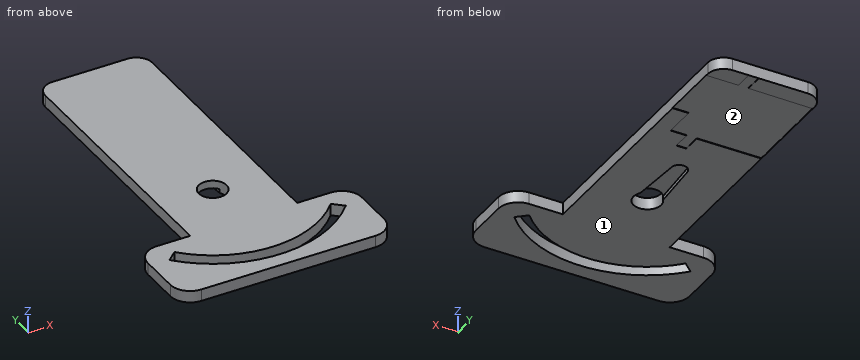
```python
from build123d import *

# Parameters (mm, degrees)
CORTE_EXTERIOR_R        = 3.500001168
SALIENTE_EXTRUIR1_DEPTH = 3
CORTAR_EXTRUIR1_DEPTH   = 1
CORTAR_EXTRUIR2_DEPTH   = 0.1


with BuildPart() as part:
    # Corte exterior → Saliente-Extruir1 (new body)
    with BuildSketch(Plane.XY):
        with BuildLine():
            Line((19.521996462, -6.085833738), (11.021996462, -6.085833738))
            ThreePointArc((11.021996462, -6.085833738), (7.486462556, -7.550299832), (6.021996462, -11.085833738))
            Line((6.021996462, -11.085833738), (6.021996462, -21.085833738))
            ThreePointArc((6.021996462, -21.085833738), (7.486462556, -24.621367644), (11.021996462, -26.085833738))
            Line((11.021996462, -26.085833738), (55.021996462, -26.085833738))
            ThreePointArc((55.021996462, -26.085833738), (58.557530368, -24.621367644), (60.021996462, -21.085833738))
            Line((60.021996462, -21.085833738), (60.021996462, -11.085833738))
            ThreePointArc((60.021996462, -11.085833738), (58.557530368, -7.550299832), (55.021996462, -6.085833738))
            Line((55.021996462, -6.085833738), (46.514841363, -6.085833738))
            Line((46.514841363, -6.085833738), (46.521996462, 58.812041738))
            ThreePointArc((46.521996462, 58.812041738), (45.350423587, 61.640468863), (42.521996462, 62.812041738))
            Line((42.521996462, 62.812041738), (23.521996462, 62.812041738))
            ThreePointArc((23.521996462, 62.812041738), (20.693569337, 61.640468863), (19.521996462, 58.812041738))
            Line((19.521996462, 58.812041738), (19.521996462, -6.085833738))
        make_face()
        with Locations((33.021996462, 7.812041474)):
            Circle(CORTE_EXTERIOR_R, mode=Mode.SUBTRACT)
        with BuildLine():
            Line((55.29494797, -12.330366391), (52.77320204, -10.049840692))
            ThreePointArc((52.77320204, -10.049840692), (33.021996462, -18.817961696), (13.270789317, -10.049842109))
            Line((13.270789317, -10.049842109), (10.749043386, -12.330367808))
            ThreePointArc((10.749043386, -12.330367808), (33.021996462, -22.217961696), (55.29494797, -12.330366391))
        make_face(mode=Mode.SUBTRACT)
    extrude(amount=SALIENTE_EXTRUIR1_DEPTH)

    # Grabado Superficie → Cortar-Extruir1 (cut)
    with BuildSketch(Plane.XY):
        with BuildLine():
            Line((35.89134848, 9.816243852), (35.017032688, 22.202862127))
            ThreePointArc((35.017032688, 22.202862127), (33.021996462, 24.062041474), (31.026960236, 22.202862127))
            Line((31.026960236, 22.202862127), (30.152644444, 9.816243852))
            ThreePointArc((30.152644444, 9.816243852), (33.021996462, 11.312042642), (35.89134848, 9.816243852))
        make_face()
    extrude(amount=CORTAR_EXTRUIR1_DEPTH, mode=Mode.SUBTRACT)

    # grabado linea medio → Cortar-Extruir2 (cut)
    with BuildSketch(Plane.XY):
        Polygon((42.460122518, 43.017187336), (46.540121977, 43.015086813), (46.547921712, 58.165084805), (38.407922791, 58.169275554), (38.41031162, 62.809274939), (35.890311954, 62.810572321), (35.887922498, 58.169356436), (19.547821697, 57.977768849), (19.535965697, 34.948988401), (35.875963531, 34.940576014), (35.873574702, 30.300576629), (38.393574368, 30.299279247), (38.395963198, 34.939278632), (42.455962659, 34.937188407), align=None)
    extrude(amount=CORTAR_EXTRUIR2_DEPTH, mode=Mode.SUBTRACT)


solid = part.part
```
Could you check a few things on this model? Use its own coordinates, in mm. Face numbers are marked on the shaded views. Coordinates: 2 decimals unless noted, no trailing zeros. Write each loop counter-clockwise with the first axis right and the second up, starting at its lowest first coordinate (ties: lowest second). Pieces come first, ordered by that corner, then holes. Notation, with made-up numbers: M -20.75,-39 L 36.25,-39 A24 cw 36.25,-1 Z; hole C 9,41 d4. An arc over 180 degrees is marked long. Answer as CSV lines item,"result". Start each with the question number.
1) We'd pull the mould along X, two halves only. Please class the marked faces 1 and 2: +X half, -X half, draft (parallel to the pull), parting line (faces both ways), or undercut.
2) For P1, Ø1.5, axis at y = -7.5, z = 2.5, coming from the +X side; P2, Ø0.9, axis at x = 17, z = 1.5, coming from the +Y side; P3, Ø4, axis at x = 29.5, y = 52, coming from the -Z side, each with a flat end and sliding along its axis, tell me the tip position at first contact or that it passes through.
3) Please list where these lines run through material, in increasing order: line 1 (X direction, y = -11, z = 1.55); line 2 (Y direction, x = 31.5, z = 1.75); line 3 (X direction, y = -14, z = 1.25). Write a range as from..to.
4) I want a section at A-A, the plane z = 0.55. Please give me the cut outline in (x, y).
5) I want a section at B-B, the plane y = 6. Please give me the cut outline in (x, z).
6) I want a section at D-D, the plane y = 16. Please give me the cut outline in (x, z).
7) I want a section at C-C, the plane y = -14. Please give me the cut outline in (x, z), and give its area (3 significant figures).
Data:
1,face 1,"draft"
1,face 2,"undercut"
2,P1,"stops at x = 59.14"
2,P2,"stops at y = -6.09"
2,P3,"stops at z = 0.1"
3,line 1,"x = 6.02..12.22, 14.17..51.87, 53.82..60.02"
3,line 2,"y = -26.09..-22.18, -18.77..4.66, 10.96..62.81"
3,line 3,"x = 6.02..12.38, 17.74..48.3, 53.66..60.02"
4,outline,"M 6.02,-21.09 A5 ccw 11.02,-26.09 L 55.02,-26.09 A5 ccw 60.02,-21.09 L 60.02,-11.09 A5 ccw 55.02,-6.09 L 46.51,-6.09 L 46.52,58.81 A4 ccw 42.52,62.81 L 23.52,62.81 A4 ccw 19.52,58.81 L 19.52,-6.09 L 11.02,-6.09 A5 ccw 6.02,-11.09 Z; hole M 10.75,-12.33 A30.03 ccw 55.29,-12.33 L 52.77,-10.05 A26.63 cw 13.27,-10.05 Z; hole M 30.15,9.82 A3.5 ccw long 35.89,9.82 L 35.02,22.2 A2 ccw 31.03,22.2 Z"
5,outline,"M 19.52,0 L 30.03,0 L 30.03,3 L 19.52,3 Z; M 36.02,0 L 46.52,0 L 46.52,3 L 36.02,3 Z"
6,outline,"M 19.52,0 L 30.59,0 L 30.59,1 L 35.45,1 L 35.45,0 L 46.52,0 L 46.52,3 L 19.52,3 Z"
7,outline,"M 6.02,0 L 12.38,0 L 12.38,3 L 6.02,3 Z; M 17.74,0 L 48.3,0 L 48.3,3 L 17.74,3 Z; M 53.66,0 L 60.02,0 L 60.02,3 L 53.66,3 Z"
7,area,"130 mm^2"
